Part model, mm, in its own coordinate system. A direction names the side the tool comes from. Coordinates: 2 decimals unless noted, no trailing zeros. Order: outer loops, then holes, each group sorted by start corner. A loop starts at its lowest first (then second) coordinate and runs counter-clockwise, first axis right, second up.
```python
from build123d import *

# Parameters (mm, degrees)
SKETCH003_R      = 3
EXTRUDE003_DEPTH = 10
EXTRUDE002_DEPTH = 5
FACE001_R        = 7
EXTRUDE001_DEPTH = 3.25
FACE_W           = 31
FACE_H           = 29
EXTRUDE_DEPTH    = 3.25
FILLET_R         = 2.1


with BuildPart() as extrude003:
    # Sketch003 (on Face19 of Cut) → Extrude003 (new body)
    with BuildSketch(Plane.XY.offset(1.5)):
        with Locations((14.5, 15.5)):
            Circle(SKETCH003_R)
    extrude(amount=-EXTRUDE003_DEPTH)


with BuildPart() as extrude002:
    # Face002 → Extrude002 (new body)
    with BuildSketch(Plane(origin=(14.5, 15.5, 6.5), x_dir=(0, 1, 0), z_dir=(0, 0, 1))):
        Polygon((-2.886751, -5), (2.886751, -5), (5.773503, 0), (2.886751, 5), (-2.886751, 5), (-5.773503, 0), align=None)
    extrude(amount=-EXTRUDE002_DEPTH)


with BuildPart() as extrude001:
    # Face001 → Extrude001 (new body)
    with BuildSketch(Plane(origin=(14.5, 15.5, 3.25), x_dir=(0, 1, 0), z_dir=(0, 0, 1))):
        Circle(FACE001_R)
    extrude(amount=EXTRUDE001_DEPTH)


with BuildPart() as cut001:
    # Face → Extrude (new body)
    with BuildSketch(Plane(origin=(14.5, 15.5, 0), x_dir=(0, 1, 0), z_dir=(0, 0, 1))):
        Rectangle(FACE_W, FACE_H)
    extrude(amount=EXTRUDE_DEPTH)

    # Fillet
    fillet_edges = [cut001.edges().sort_by_distance(p)[0] for p in [
        (0, 0, 1.625),
        (29, 0, 1.625),
        (29, 31, 1.625),
        (0, 31, 1.625),
    ]]
    fillet(fillet_edges, radius=FILLET_R)

    # Fusion: union Extrude001
    add(extrude001.part)

    # Cut: cut Extrude002
    add(extrude002.part, mode=Mode.SUBTRACT)

    # Cut001: cut Extrude003
    add(extrude003.part, mode=Mode.SUBTRACT)


solid = cut001.part
```
(1) Slice it at D-D, the plane y = 19. Give the cut face in (x, z), then the cut area to 3 significant figures.
(2) Drop a flat-ended pin along its axis: pin 1 (7 mm diameter, centred on x = 14.5, y = 15.5, fed in from -Z). Give the stop position or say it passes through.
(3) Probe line 1 (Y direction, x = 14.5, z = 0.95); line 2 (Z direction, x = 25, y = 7); line 3 (Z direction, x = 15.75, y = 19.5). List the from-to ranges inside material, lowest first.
(4) Slice it at C-C, the plane x = 12.5. Give the cut face in (y, z).
(5) Slice it at A-A, the plane z = 2.25. Give the cut face in (x, y).
(6) Tool access for faces 1 (the face through (0.63, 0.6, 1.65)), 2 (the face through (17.035, 19.81, 4.035)): list every direction of +Z, -Z, +X, -X, +Y, -Y with a clear straight run to the whole face (end or side of a thin tool).
(7) Pull direction X, two halves, no side cores. Call faces 3 (the face through (15, 0, 2)), 4 (the face through (12, 18, 1.5)), 5 (the face through (28.37, 0.6, 1.65)): +X half, -X half, draft (parallel to the pull), parting line (faces both ways), or undercut.
(8) Slice it at B-B, the plane y = 15.5. Give the cut face in (x, z), then the cut area to 4 significant figures.
Here are the results:
1. outline: (0, 0) - (29, 0) - (29, 3.25) - (20.56, 3.25) - (20.56, 6.5) - (18.44, 6.5) - (18.44, 1.5) - (10.56, 1.5) - (10.56, 6.5) - (8.44, 6.5) - (8.44, 3.25) - (0, 3.25) - close
1. area: 94.3 mm2
2. pin 1: stops at z = 0
3. line 1: y = 0 to 12.5, 18.5 to 31
3. line 2: z = 0 to 3.25
3. line 3: z = 0 to 1.5
4. outline: (0, 0) - (13.26, 0) - (13.26, 1.5) - (10.88, 1.5) - (10.88, 6.5) - (8.79, 6.5) - (8.79, 3.25) - (0, 3.25) - close; (17.74, 0) - (31, 0) - (31, 3.25) - (22.21, 3.25) - (22.21, 6.5) - (20.12, 6.5) - (20.12, 1.5) - (17.74, 1.5) - close
5. outline: (0, 2.1) arc R2.1 ccw to (2.1, 0) - (26.9, 0) arc R2.1 ccw to (29, 2.1) - (29, 28.9) arc R2.1 ccw to (26.9, 31) - (2.1, 31) arc R2.1 ccw to (0, 28.9) - close; hole (9.5, 12.61) - (14.5, 9.73) - (19.5, 12.61) - (19.5, 18.39) - (14.5, 21.27) - (9.5, 18.39) - close
6. face 1: +Z, -Z, -X, -Y
6. face 2: +Z
7. face 3: draft
7. face 4: undercut
7. face 5: +X half
8. outline: (0, 0) - (11.5, 0) - (11.5, 1.5) - (9.5, 1.5) - (9.5, 6.5) - (7.5, 6.5) - (7.5, 3.25) - (0, 3.25) - close; (17.5, 0) - (29, 0) - (29, 3.25) - (21.5, 3.25) - (21.5, 6.5) - (19.5, 6.5) - (19.5, 1.5) - (17.5, 1.5) - close
8. area: 80.75 mm2
